Read the model definition and answer for the solid it produces. Units are mm, in the model's axes. A direction names the side the tool comes from. Coordinates: 2 decimals unless noted, no trailing zeros. Write each loop counter-clockwise with the first axis right and the second up, starting at its lowest first coordinate (ties: lowest second). Pieces come first, ordered by that corner, then holes.
1) The part is cut by section C-C (y = 12.5). Determine the outline of the cut face in (x, z).
2) The part is cut by section D-D (y = 19.75). Determine the outline of the cut face in (x, z), then the cut area to 3 significant figures.
3) Each of these flat-tipped pins is pushed along its axis until it touches: pin 1 Ø12 at (x, y) = (11, 17.5) entering from -Z; pin 2 Ø5 at (y, z) = (8, -8.5) entering from -X; pin 3 Ø2.5 at (x, y) = (7, 16) entering from -Z. Where does it stop, or does it pass through?
4) The part is cut by section B-B (x = 26.5). Determine the outline of the cut face in (y, z), then the cut area to 3 significant figures.
5) Which of the six approach directions +Z, -Z, +X, -X, +Y, -Y give full straight-line access (tool end or side, diameter ignored) to faces 1 (the face through (10.094, 12, -6)), 2 (the face through (38, 12, -1.113)), 3 (the face through (17, 0, -4))?
6) Determine the mould class of faces 4 (the face through (21.1, 12.32, -22.36)), 5 (the face through (22, 12, 3.887)), 6 (the face through (32.594, 12, -6)), 7 (the face through (18.38, 12.32, -3.95)) for opening direction Z: +Z half, -Z half, draft (parallel to the pull), parting line (faces both ways), or undercut.
7) The part is cut by section A-A (z = -13.5). Determine the outline of the cut face in (x, y), then the cut area to 3 significant figures.
8) Find the intervals of material crossed by line 1 (X direction, y = 14.5, z = -6.25); line 2 (Z direction, x = 6.5, y = 15.25); line 3 (X direction, y = 23.5, z = -6), in increasing order.
from build123d import *

# Parameters (mm, degrees)
SKETCH_1_R          = 7.75
EXTRUDE_1_DEPTH     = 25
SKETCH_2_R          = 1.75
CUT_EXTRUDE_1_DEPTH = 53.781587215


with BuildPart() as part:
    # 草图1 → 凸台-拉伸1 (new body)
    with BuildSketch(Plane(origin=(0, 0, 0), x_dir=(1, 0, 0), z_dir=(0, 1, 0))):
        with BuildLine():
            Line((1.344086022, 1.112903226), (10.094086022, 1.112903226))
            Line((10.094086022, 1.112903226), (10.094086022, 11.112903226))
            ThreePointArc((10.094086022, 11.112903226), (21.344086022, 22.362903226), (32.594086022, 11.112903226))
            Line((32.594086022, 11.112903226), (32.594086022, 1.112903226))
            Line((32.594086022, 1.112903226), (41.344086022, 1.112903226))
            Line((41.344086022, 1.112903226), (41.344086022, -3.887096774))
            Line((41.344086022, -3.887096774), (1.344086022, -3.887096774))
            Line((1.344086022, -3.887096774), (1.344086022, 1.112903226))
        make_face()
        with Locations(Location((21.344086022, 11.112903226, 0), (0, 0, 270))):
            Circle(SKETCH_1_R, mode=Mode.SUBTRACT)
    extrude(amount=EXTRUDE_1_DEPTH)

    # 草图2 → 切除-拉伸1 (cut, through all)
    with BuildSketch(Plane(origin=(0, 0, -1.112903226), x_dir=(-1, 0, 0), z_dir=(0, 0, -1))):
        with Locations((-35.344086022, 12.5)):
            Circle(SKETCH_2_R)
        with Locations((-7.344086022, 12.5)):
            Circle(SKETCH_2_R)
    extrude(amount=-CUT_EXTRUDE_1_DEPTH, mode=Mode.SUBTRACT)


solid = part.part
Reported:
1. outline: (1.34, -1.11) - (5.59, -1.11) - (5.59, 3.89) - (1.34, 3.89) - close; (9.09, -1.11) - (10.09, -1.11) - (10.09, -11.11) arc R11.25 ccw to (32.59, -11.11) - (32.59, -1.11) - (33.59, -1.11) - (33.59, 3.89) - (9.09, 3.89) - close; (37.09, -1.11) - (41.34, -1.11) - (41.34, 3.89) - (37.09, 3.89) - close; hole circle Ø15.5 at (21.34, -11.11)
2. outline: (1.34, -1.11) - (10.09, -1.11) - (10.09, -11.11) arc R11.25 ccw to (32.59, -11.11) - (32.59, -1.11) - (41.34, -1.11) - (41.34, 3.89) - (1.34, 3.89) - close; hole circle Ø15.5 at (21.34, -11.11)
2. area: 435 mm2
3. pin 1: stops at z = -21.49
3. pin 2: stops at x = 10.09
3. pin 3: stops at z = -1.11
4. outline: (0, -21.11) - (25, -21.11) - (25, -16.9) - (0, -16.9) - close; (0, -5.33) - (25, -5.33) - (25, 3.89) - (0, 3.89) - close
4. area: 336 mm2
5. face 1: -Z, -X, +Y, -Y
5. face 2: -Z, +X, +Y, -Y
5. face 3: +Z, -Z, +X, -X, -Y
6. face 4: -Z half
6. face 5: +Z half
6. face 6: draft
6. face 7: undercut
7. outline: (10.35, 0) - (13.97, 0) - (13.97, 25) - (10.35, 25) - close; (28.72, 0) - (32.34, 0) - (32.34, 25) - (28.72, 25) - close
7. area: 181 mm2
8. line 1: x = 10.09 to 15.31, 27.38 to 32.59
8. line 2: z = -1.11 to 3.89
8. line 3: x = 10.09 to 15.52, 27.17 to 32.59
